The drawing under review shows one solid part. Ordinate dimensions are in mm from its lowest x, y, z. Round coordinates to 2 decimals unless told otherwise and drop trailing zeros. Write each loop counter-clockwise with the first axis right and the second up, starting at its lowest first coordinate (ties: lowest second). Pieces come first, ordered by that corner, then holes. Notation, with made-up numbers: M -28,-10.5 L 18,-10.5 A5 cw 18,-1.5 Z; hole C -39.75,-30 d6. An arc over 180 degrees is marked long. One line per item, written item: value. Start each with the question number.
1) For P1, Ø6, axis at x = 58, z = 361.5, coming from the -Y side (1 decimal); P2, Ø12, axis at y = 23.5, z = 555.5, coming from the -X side; P3, Ø8, axis at y = 27.5, z = 104, coming from the -X side; P4, Ø5, axis at y = 37, z = 785, coming from the -X side, all flat-tipped, find the tip position at first contact; note any pin that passes through.
2) Wall thickness on probe 1 along Z at (x, y) = (15, 47); probe 2 along X at (y, z) = (29.5, 259.5); probe 3 along X at (y, z) = (35, 468) (1 decimal): over which ranges is each line inside the solid? List them lowest first.
3) Take a section at A-A, the plane z = 326. Write out the cut boundary in (x, y).
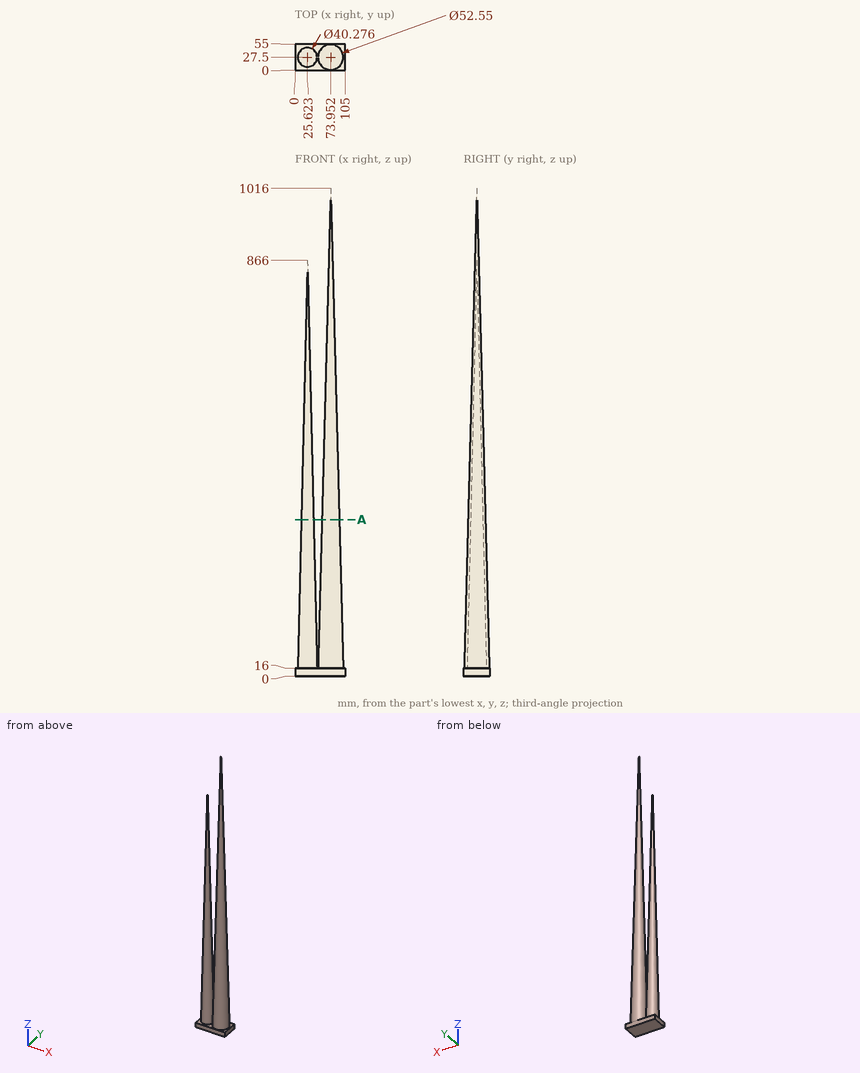
Checked values:
1. P1: stops at y = 16.2
1. P2: stops at x = 18.16
1. P3: stops at x = 7.48
1. P4: passes through
2. probe 1: z = 0 to 16
2. probe 2: x = 11.39 to 39.85, 54.18 to 93.73
2. probe 3: x = 19.9 to 31.3, 61.7 to 86.2
3. outline: C 25.62,27.5 d25.59; C 73.95,27.5 d36.26
